Part model, mm, in its own coordinate system. A direction names the side the tool comes from. Round coordinates to 2 decimals unless told otherwise and drop trailing zeros. Write each loop counter-clockwise with the first axis right and the second up, starting at its lowest first coordinate (ties: lowest second). Pieces come first, ordered by that corner, then holes. Notation, with made-up numbers: (19.5, 66.25) -> (54.5, 66.25) arc R24 ccw to (54.5, 98.25) -> close; hole circle Ø2 at (1.25, -7). An arc over 180 degrees is marked (long way). Use CSV: the item, a comma, the result in double quotes. Start each with the question number.
(1) Drop a flat-ended pin along its axis: pin 1 (4 mm diameter, centred on x = -15.5, z = -20, fed in from +Y). Give the stop position or say it passes through.
(2) Saw through at A-A (z = -16). Give the cut face in (x, y) (3 decimals), plus the area to 3 significant figures.
(3) Saw through at C-C (y = -1.9). Count the separate pieces of the cut face and the enclosed holes in it, plus the area to 3 significant figures.
(4) Two-plate mould, pull along Z, no slides. Class faces 1 (the cylindrical face through (16.013, -1.565, 9.181)), 2 (the flat face through (-1, -2, -33.338)), 3 (the flat face through (-1, -2, 33.338)): released by +Z, released by -Z, zero draft, split by the parting line, or undercut.
(5) Saw through at B-B (x = -13.5). Give the cut face in (y, z) (1 decimal).
(6) Which spindle directions (+Z, -Z, +X, -X, +Y, -Y) get a long thin tool onto all of the face, cutting with end or side? Do faces 4 (the flat face through (-1, 0, 0)), 5 (the flat face through (-15, -2, 11.112)). Say none if no direction does.
(7) Probe line 1 (X direction, y = -0.8, z = 1); line 2 (X direction, y = -1.2, z = -9); line 3 (Z direction, x = -18.5, y = -1.55). List the from-to ranges inside material, lowest first. Write a range as [from, to].
```python
from build123d import *

# Parameters (mm, degrees)
F0_W     = 77.7875
F0_H     = 66.675
F1_DEPTH = 3.175
F3_D     = 6.35
F5_D     = 6.35
F6_W     = 12.7
F6_H     = 15.875
F7_DEPTH = 3.176


with BuildPart() as f1:
    # F0 (on Front) → F1 (new body)
    with BuildSketch(Plane.XZ):
        Rectangle(F0_W, F0_H)
    extrude(amount=F1_DEPTH)

    # F3 (through all)
    with Locations(Plane.XZ.offset(3.175)):
        with Locations((-15.08125, -11.1125)):
            Hole(F3_D / 2)

    # F5 (through all)
    with Locations(Plane.XZ.offset(3.175)):
        with Locations((13.49375, 11.1125)):
            Hole(F5_D / 2)

    # F6 (on face) → F7 (cut, through all)
    with BuildSketch(Plane.XZ.offset(3.175)):
        with Locations((-15.08125, 3.175)):
            Rectangle(F6_W, F6_H)
        with Locations((11.90625, -11.1125)):
            Rectangle(F6_W, F6_H)
    extrude(amount=-F7_DEPTH, mode=Mode.SUBTRACT)


solid = f1.part
```
Answers:
1,pin 1,"stops at y = 0"
2,outline,"(-38.894, -3.175) -> (5.556, -3.175) -> (5.556, 0) -> (-38.894, 0) -> close; (18.256, -3.175) -> (38.894, -3.175) -> (38.894, 0) -> (18.256, 0) -> close"
2,area,"207 mm²"
3,separate pieces,"1"
3,enclosed holes,"4"
3,area,"4,720 mm²"
4,face 1,"undercut"
4,face 2,"released by -Z"
4,face 3,"released by +Z"
5,outline,"(-3.2, -33.3) -> (0, -33.3) -> (0, -13.9) -> (-3.2, -13.9) -> close; (-3.2, -8.4) -> (0, -8.4) -> (0, -4.8) -> (-3.2, -4.8) -> close; (-3.2, 11.1) -> (0, 11.1) -> (0, 33.3) -> (-3.2, 33.3) -> close"
6,face 4,"+Z, -Z, +X, -X, +Y"
6,face 5,"+Y, -Y"
7,line 1,"x = [-38.89, -21.43], [-8.73, 38.89]"
7,line 2,"x = [-38.89, -17.45], [-12.71, 5.56], [18.26, 38.89]"
7,line 3,"z = [-33.34, -4.76], [11.11, 33.34]"
